Source: CAD feature listing. Evaluate the final solid. Frame: model axes, mm. Coordinates: 2 decimals unless noted, no trailing zeros. Write each loop counter-clockwise with the first axis right and the second up, starting at its lowest first coordinate (ties: lowest second). Pieces come first, ordered by that corner, then holes. Notation, with made-up numbers: M 2.25,63.25 L 18.25,63.25 A19 cw 18.25,74.25 Z; hole C 18,39 d8. An arc over 180 degrees is marked long. Answer as CSV lines item,"result". Start each with the question number.
1. Section D-D on z = 11.25. Return the cut outline in (x, y) (3 decimals).
2. Section A-A on x = 0. Return the cut outline in (y, z) (3 decimals).
3. Section C-C on z = 0. Return the cut outline in (x, y) (3 decimals).
4. Line query: probe 1 along X at (y, z) = (2.2, 15); probe 2 along X at (y, z) = (1.6, 0); probe 3 along X at (y, z) = (0.7, 11.25). Output: solid intervals per line, ascending. Write a range as [from, to].
5. Contact query for flat-ended pins moving along their axis: pin 1 Ø5 at (x, z) = (-22, -0.5) entering from +Y (3 decimals); pin 2 Ø6 at (x, z) = (0, 0) entering from -Y; pin 3 Ø1 at (x, y) = (-31, 2.5) entering from +Z. Output: stop coordinate, or through.
6. Section B-B on z = -27. Return the cut outline in (x, y) (3 decimals), plus the area to 3 significant figures.
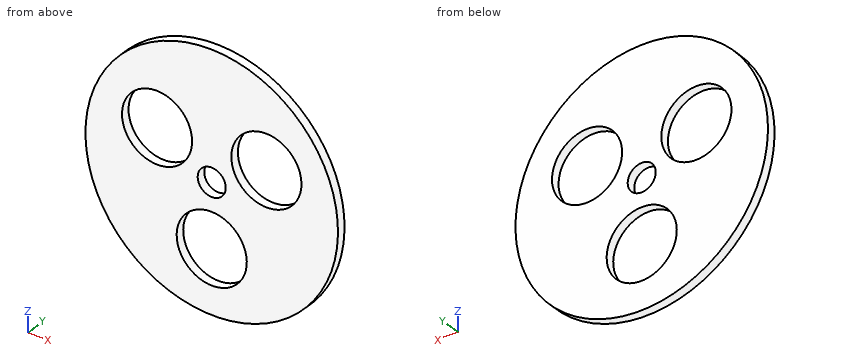
```python
from build123d import *

# Parameters (mm, degrees)
SKETCH1_R           = 45
SKETCH1_R_2         = 12.5
BOSS_EXTRUDE1_DEPTH = 3.175
SKETCH3_R           = 5
CUT_EXTRUDE1_DEPTH  = 6.35


with BuildPart() as part:
    # Sketch1 → Boss-Extrude1 (new body)
    with BuildSketch(Plane(origin=(0, 0, 0), x_dir=(1, 0, 0), z_dir=(0, 1, 0))):
        with Locations(Location((0, 0, 0), (0, 0, 270))):
            Circle(SKETCH1_R)
        with Locations(Location((0, 22.5, 0), (0, 0, 270))):
            Circle(SKETCH1_R_2, mode=Mode.SUBTRACT)
        with Locations(Location((19.485571585, -11.25, 0), (0, 0, 270))):
            Circle(SKETCH1_R_2, mode=Mode.SUBTRACT)
        with Locations(Location((-19.485571585, -11.25, 0), (0, 0, 270))):
            Circle(SKETCH1_R_2, mode=Mode.SUBTRACT)
    extrude(amount=BOSS_EXTRUDE1_DEPTH)

    # Sketch3 → Cut-Extrude1 (cut)
    with BuildSketch(Plane(origin=(0, 3.175, 0), x_dir=(1, 0, 0), z_dir=(0, 1, 0))):
        with Locations(Location((0, 0, 0), (0, 0, 270))):
            Circle(SKETCH3_R)
    extrude(amount=-CUT_EXTRUDE1_DEPTH, mode=Mode.SUBTRACT)


solid = part.part
```
Values:
1,outline,"M -43.571,0 L -31.986,0 L -31.986,3.175 L -43.571,3.175 Z; M -6.986,0 L 6.986,0 L 6.986,3.175 L -6.986,3.175 Z; M 31.986,0 L 43.571,0 L 43.571,3.175 L 31.986,3.175 Z"
2,outline,"M 0,-45 L 3.175,-45 L 3.175,-35 L 0,-35 Z; M 0,-10 L 3.175,-10 L 3.175,-5 L 0,-5 Z; M 0,5 L 3.175,5 L 3.175,45 L 0,45 Z"
3,outline,"M -45,0 L -24.934,0 L -24.934,3.175 L -45,3.175 Z; M -14.037,0 L -5,0 L -5,3.175 L -14.037,3.175 Z; M 5,0 L 14.037,0 L 14.037,3.175 L 5,3.175 Z; M 24.934,0 L 45,0 L 45,3.175 L 24.934,3.175 Z"
4,probe 1,"[-42.43, -31.41], [-7.56, 7.56], [31.41, 42.43]"
4,probe 2,"[-45, -24.93], [-14.04, -5], [5, 14.04], [24.93, 45]"
4,probe 3,"[-43.57, -31.99], [-6.99, 6.99], [31.99, 43.57]"
5,pin 1,"y = 3.175"
5,pin 2,"through"
5,pin 3,"z = 33.09"
6,outline,"M -36,0 L -11.662,0 L -11.662,3.175 L -36,3.175 Z; M 11.662,0 L 36,0 L 36,3.175 L 11.662,3.175 Z"
6,area,"155 mm²"
